Input: part model. Units: mm. Frame: model coordinates. Face numbers are marked on the shaded views. A direction names the side the tool comes from. Round coordinates to 2 decimals unless told otherwise and drop trailing zeros. Write each loop counter-clockwise with the first axis right and the second up, starting at its lowest first coordinate (ties: lowest second). Pieces come first, ordered by that corner, then holes. Notation, with made-up numbers: (78.25, 44.25) - (116.25, 44.25) arc R21 cw to (116.25, 54.25) - close; hole circle Ø2 at (-19, -2.75). An arc over 180 degrees is marked (long way). Use one line per item in the form item = value.
```python
from build123d import *

# Parameters (mm, degrees)
SKETCH_R        = 12
PAD_DEPTH       = 40
SKETCH001_W     = 75.633354
SKETCH001_H     = 46.920013
POCKET_DEPTH    = 55
SKETCH002_W     = 41.400021
SKETCH002_H     = 16
POCKET001_DEPTH = 8
SKETCH003_W     = 67.968546
SKETCH003_H     = 93.61967
POCKET002_DEPTH = 40
POCKET003_DEPTH = 28.001


with BuildPart() as part:
    # Sketch → Pad (new body, symmetric)
    with BuildSketch(Plane.XZ):
        with BuildLine():
            Line((-40, 32), (29, 32))
            ThreePointArc((44, 17), (39.606602, 27.606602), (29, 32))
            Line((44, 17), (44, -8))
            ThreePointArc((12, -40), (34.627417, -30.627417), (44, -8))
            Line((12, -40), (-40, -40))
            Line((-40, -40), (-40, 32))
        make_face()
        Circle(SKETCH_R, mode=Mode.SUBTRACT)
    extrude(amount=PAD_DEPTH, both=True)

    # Sketch001 → Pocket (cut)
    with BuildSketch(Plane.XZ.offset(40)):
        with Locations((25.816677, 23.460006)):
            Rectangle(SKETCH001_W, SKETCH001_H)
    extrude(amount=-POCKET_DEPTH, mode=Mode.SUBTRACT)

    # Sketch002 → Pocket001 (cut)
    with BuildSketch(Plane.XZ.offset(40)):
        with Locations((-28.213342, 16)):
            Rectangle(SKETCH002_W, SKETCH002_H)
    extrude(amount=-POCKET001_DEPTH, mode=Mode.SUBTRACT)

    # Sketch003 → Pocket002 (cut)
    with BuildSketch(Plane(origin=(0, 40, 0), x_dir=(1, 0, 0), z_dir=(0, 1, 0))):
        with Locations((-21.984273, 2.649843)):
            Rectangle(SKETCH003_W, SKETCH003_H)
    extrude(amount=-POCKET002_DEPTH, mode=Mode.SUBTRACT)

    # Sketch004 → Pocket003 (cut, through all)
    with BuildSketch(Plane(origin=(-12, 0, 0), x_dir=(0, 0, 1), z_dir=(1, 0, 0))):
        Polygon((32, 12), (32, 0), (7, 0), align=None)
    extrude(amount=-POCKET003_DEPTH, mode=Mode.SUBTRACT)


solid = part.part
```
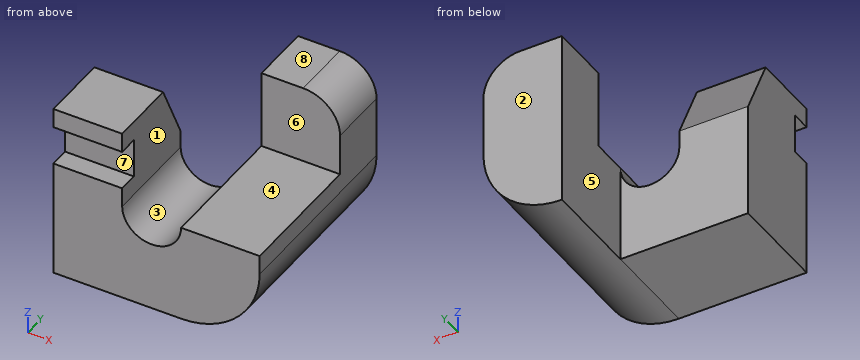
(1) First-contact query: pin 1 Ø8 at (y, z) = (-11.5, 18) entering from +X; pin 2 Ø2 at (x, z) = (-26.5, 20.5) entering from -Y; pin 3 Ø1 at (x, y) = (20, -29.5) entering from +Z. Flat tips, straight axial feed; report the tip coordinate or a pass-through.
Derived:
pin_1 = -12
pin_2 = -32
pin_3 = 0
(2) Cut plane C-C on x = -19. Output: boundary loops of the cut face in (y, z), then the cut area to 3 significant figures.
Derived:
outline = (-40, -40) - (0, -40) - (0, 7) - (-12, 32) - (-40, 32) - (-40, 24) - (-32, 24) - (-32, 8) - (-40, 8) - close
area = 2,600 mm^2
(3) Material intervals for L1, parallel to X at y = -7.5, z = 21; L2, parallel to X at y = -22, z = -7; L3, parallel to Y at x = -31, z = -18, sorted ascending.
Derived:
L1 = -40 to -12
L2 = -40 to -9.75, 9.75 to 44
L3 = -40 to 0
(4) Draft query along X for the marked faces 1, 2 and 3. Return one class per face: released by +X, released by -X, zero draft, split by the parting line, or undercut.
Derived:
face_1 = released by +X
face_2 = zero draft
face_3 = undercut
(5) Cut plane D-D on z = 1.5. Output: boundary loops of the cut face in (x, y), then the cut area to 3 significant figures.
Derived:
outline = (-40, -40) - (-12, -40) - (-12, 0) - (-40, 0) - close; (12, 15) - (44, 15) - (44, 40) - (12, 40) - close
area = 1,920 mm^2
(6) Cut plane A-A on z = 10. Output: boundary loops of the cut face in (x, y), then the cut area to 3 significant figures.
Derived:
outline = (-40, -32) - (-12, -32) - (-12, -1.44) - (-40, -1.44) - close; (12, 15) - (44, 15) - (44, 40) - (12, 40) - close
area = 1,660 mm^2
(7) Cut plane B-B on y = -26. Output: boundary loops of the cut face in (x, z), then the cut area to 3 significant figures.
Derived:
outline = (-40, -40) - (12, -40) arc R32 ccw to (44, -8) - (44, 0) - (12, 0) arc R12 cw to (-12, 0) - (-12, 32) - (-40, 32) - close
area = 3,810 mm^2
(8) Access query for the marked faces 4, 5, 6, 7 and 8. Directions: +Z, -Z, +X, -X, +Y, -Y. A direction counts if a zero-diameter tool reaches every point of the face in a straight line with its end or side. Return the directions, or none.
Derived:
face_4 = +Z, +X, -Y
face_5 = +Z, -Z, -X, +Y
face_6 = +Z, +X, -X, -Y
face_7 = +X, -X, -Y
face_8 = +Z, +X, -X, +Y, -Y
